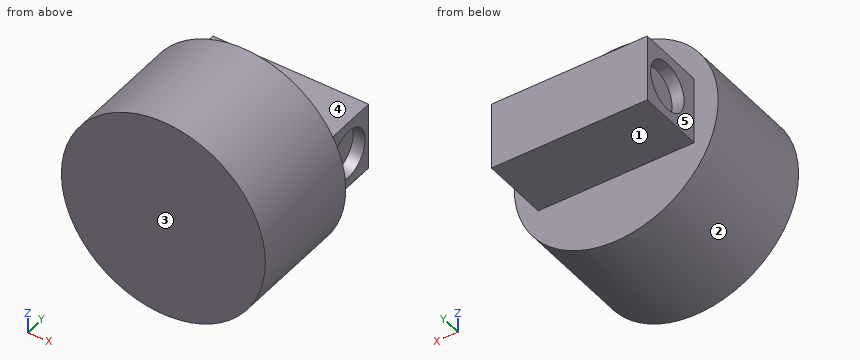
from build123d import *

# Parameters (mm, degrees)
SKETCH1_R           = 42.15
BOSS_EXTRUDE1_DEPTH = 48
SKETCH2_W           = 64.43
SKETCH2_H           = 28
BOSS_EXTRUDE2_DEPTH = 28
SKETCH3_R           = 10
CUT_EXTRUDE1_DEPTH  = 5


with BuildPart() as part:
    # Sketch1 → Boss-Extrude1 (new body)
    with BuildSketch(Plane(origin=(0, 0, 0), x_dir=(1, 0, 0), z_dir=(0, 1, 0))):
        with Locations((0, 5.951400749)):
            Circle(SKETCH1_R)
    extrude(amount=BOSS_EXTRUDE1_DEPTH)

    # Sketch2 → Boss-Extrude2 (add)
    with BuildSketch(Plane(origin=(0, 48, 0), x_dir=(1, 0, 0), z_dir=(0, 1, 0))):
        with Locations((0, 5.951400749)):
            Rectangle(SKETCH2_W, SKETCH2_H)
    extrude(amount=BOSS_EXTRUDE2_DEPTH)

    # Sketch3 → Cut-Extrude1 (cut)
    with BuildSketch(Plane.ZY.offset(32.215)):
        with Locations((-5.951400749, 64)):
            Circle(SKETCH3_R)
    cut_extrude1 = extrude(amount=-CUT_EXTRUDE1_DEPTH, mode=Mode.SUBTRACT)

    # Mirror2: Cut-Extrude1 across plane
    add(cut_extrude1.mirror(Plane.ZY), mode=Mode.SUBTRACT)


solid = part.part
Model file for the job. Use its own axes, mm. Face numbers are marked on the shaded views. A direction names the side the tool comes from. Coordinates: 2 decimals unless noted, no trailing zeros. Loops run counter-clockwise (first coordinate to the right, second up) from the corner with the lowest first, then second, coordinate; pieces in that order, holes last. Notation, with made-up numbers: (82, -21) -> (125, -21) arc R21 ccw to (125, -13) -> close; hole circle Ø4 at (63, 10). An arc over 180 degrees is marked (long way). Use one line per item in the form item = value. Start each with the question number.
(1) Cut at C-C on y = 64. Give the cut face in (x, z) (3 decimals), and give its area (3 significant figures).
(2) Probe probe 1 along Y at (x, z) = (-12.5, 16); probe 2 along Z at (x, y) = (16, 49.5); probe 3 along X at (y, z) = (52, 6.5) (3 decimals). List the from-to ranges inside material, lowest first. Write a range as from..to.
(3) Cut at A-A on x = 0. Give the cut face in (y, z).
(4) Tool access for the marked faces 1, 2, 3, 4 and 5: list every direction of +Z, -Z, +X, -X, +Y, -Y with a clear straight run to the whole face (end or side of a thin tool).
(5) Cut at B-B on z = -8.5. Give the cut face in (x, y) (3 decimals).
(6) Flat gauge pins, fed straight in: pin 1 (3 mm diameter, centred on x = -12.5, y = 9.5, fed in from +Z); pin 2 (22.5 mm diameter, centred on y = 57.5, z = -8.5, fed in from -X); pin 3 (16 mm diameter, centred on y = 64, z = -5.95, fed in from +X) (3 decimals); pin 4 (5 mm diameter, centred on x = 16, z = 16, fed in from +Y). Where does each tip first touch, or does it go through?
(7) Cut at D-D on x = -9. Give the cut face in (y, z), and give its area (3 significant figures).
Values:
q1.outline = (-32.215, -19.951) -> (32.215, -19.951) -> (32.215, -15.951) -> (27.215, -15.951) -> (27.215, 4.049) -> (32.215, 4.049) -> (32.215, 8.049) -> (-32.215, 8.049) -> (-32.215, 4.049) -> (-27.215, 4.049) -> (-27.215, -15.951) -> (-32.215, -15.951) -> close
q1.area = 1,600 mm2
q2.probe_1 = 0..48
q2.probe_2 = -19.95..8.05
q2.probe_3 = -32.215..32.215
q3.outline = (0, -48.1) -> (48, -48.1) -> (48, -19.95) -> (76, -19.95) -> (76, 8.05) -> (48, 8.05) -> (48, 36.2) -> (0, 36.2) -> close
q4.face_1 = -Z, +X, -X, +Y
q4.face_2 = +Y, -Y
q4.face_3 = +Z, -Z, +X, -X, -Y
q4.face_4 = +Z, +X, -X, +Y
q4.face_5 = +Z, -Z, -X, +Y
q5.outline = (-42.073, 0) -> (42.073, 0) -> (42.073, 48) -> (32.215, 48) -> (32.215, 54.33) -> (27.215, 54.33) -> (27.215, 73.67) -> (32.215, 73.67) -> (32.215, 76) -> (-32.215, 76) -> (-32.215, 73.67) -> (-27.215, 73.67) -> (-27.215, 54.33) -> (-32.215, 54.33) -> (-32.215, 48) -> (-42.073, 48) -> close
q6.pin_1 = 34.74
q6.pin_2 = -42.15
q6.pin_3 = 27.215
q6.pin_4 = 48
q7.outline = (0, -47.13) -> (48, -47.13) -> (48, -19.95) -> (76, -19.95) -> (76, 8.05) -> (48, 8.05) -> (48, 35.23) -> (0, 35.23) -> close
q7.area = 4,740 mm2
